```python
from build123d import *

# Parameters (mm, degrees)
SKETCH_R          = 12.75
PAD_DEPTH         = 20
SKETCH001_W       = 2.064916
SKETCH001_H       = 9
POCKET_DEPTH      = 22.001
POCKET_DEPTH_BACK = 22.001


with BuildPart() as part:
    # Sketch → Pad (new body)
    with BuildSketch(Plane.XY):
        with BuildLine():
            ThreePointArc((18.2, -21.818132), (0, 0), (-18.2, -21.818132))
            ThreePointArc((-21.643243, -22.445887), (-19.607744, -23.853631), (-18.2, -21.818132))
            ThreePointArc((-14.264293, -1.750971), (-20.722154, -11.111337), (-21.643243, -22.445887))
            ThreePointArc((-14.264293, -1.750971), (-11.495515, 3.655407), (-13.352959, 9.438568))
            ThreePointArc((13.352959, 9.438568), (0, 38.25), (-13.352959, 9.438568))
            ThreePointArc((13.352959, 9.438568), (11.495515, 3.655407), (14.264293, -1.750971))
            ThreePointArc((21.643243, -22.445887), (20.722154, -11.111337), (14.264293, -1.750971))
            ThreePointArc((18.2, -21.818132), (19.607744, -23.853631), (21.643243, -22.445887))
        make_face()
        with Locations((0, 20.75)):
            Circle(SKETCH_R, mode=Mode.SUBTRACT)
    extrude(amount=PAD_DEPTH)

    # Sketch001 → Pocket (cut, two sides)
    with BuildSketch(Plane.YZ) as pocket_sk:
        with Locations((-20.667451, 10)):
            Rectangle(SKETCH001_W, SKETCH001_H)
    extrude(amount=-POCKET_DEPTH, mode=Mode.SUBTRACT)
    extrude(pocket_sk.sketch, amount=POCKET_DEPTH_BACK, mode=Mode.SUBTRACT)


solid = part.part
```
The listing builds one solid part. Answer for the finished solid, in the listing's coordinates (mm). A direction names the side the tool comes from. Round coordinates to 2 decimals unless told otherwise and drop trailing zeros. Order: outer loops, then holes, each group sorted by start corner. A loop starts at its lowest first (then second) coordinate and runs counter-clockwise, first axis right, second up. Notation, with made-up numbers: (-17, 57) - (26, 57) arc R6 cw to (26, 67) - close; hole circle Ø1 at (-35, 85). An arc over 180 degrees is marked (long way). Put each result on its own line as item: value. Start each with the question number.
(1) Determine the mould class of faces 3 (the cylindrical face through (6.854, 31.501, 9.86)), 4 (the flat face through (-2, 7, 20)), 5 (the flat face through (20, -19.635, 10)) for opening direction Y: released by +Y, released by -Y, zero draft, split by the parting line, or undercut.
(2) Given P1, Ø2, axis at y = 7.5, z = 6.5, coming from the +X side; P2, Ø5, axis at x = -17, z = 14.5, coming from the +Y side; P3, Ø2, axis at x = 6.5, z = 11, coming from the -Y side; P4, Ø2.5, axis at x = 21, y = -21, coming from the -Z side, each flat-ended and moving along its own axis, determine where each tip first touches the part or whether it passes through.
(3) Find section B-B (z = 11.75). Give the vertices of the cut face in (x, y) (3 decimals).
(4) Find section D-D (y = 7). Give the vertices of the cut face in (x, z).
(5) For faces 1 (the flat face through (20, -21, 5.5)), 2 (the cylindrical face through (-11.5, 3.6, 9.9)), determine the directions among +Z, -Z, +X, -X, +Y, -Y from which every point of the face is accessible in a straight line to the end or side of a thin tool.
(6) Straight lines are drawn through the part: probe 1 along X at (y, z) = (-18.5, 10.75); probe 2 along X at (y, z) = (-12, 16); probe 3 along Y at (x, z) = (-9, 14). For each, find the intervals that lie inside material, in ascending order. Write a range as from..to.
(7) Find section A-A (x = 0). Give the vertices of the cut face in (y, z).
(8) Find section C-C (y = -18.5). Give the vertices of the cut face in (x, z).
Reply:
1. face 3: undercut
1. face 4: zero draft
1. face 5: undercut
2. P1: x = 12.67
2. P2: y = 30.55
2. P3: y = -1.59
2. P4: z = 0
3. outline: (-21.971, -19.635) - (-18.465, -19.635) arc R18.5 cw (long way) to (18.465, -19.635) - (21.971, -19.635) arc R22 ccw to (14.264, -1.751) arc R7.949 cw to (13.353, 9.439) arc R17.5 ccw (long way) to (-13.353, 9.439) arc R7.949 cw to (-14.264, -1.751) arc R22 ccw to start; (-21.766, -21.7) arc R22 ccw to (-21.643, -22.446) arc R1.75 ccw to (-18.2, -21.818) arc R18.5 cw to (-18.221, -21.7) - close; (18.2, -21.818) arc R1.75 ccw to (21.643, -22.446) arc R22 ccw to (21.766, -21.7) - (18.221, -21.7) arc R18.5 cw to start; hole circle Ø25.5 at (0, 20.75)
4. outline: (-11.94, 0) - (11.94, 0) - (11.94, 20) - (-11.94, 20) - close
5. face 1: +X, -X
5. face 2: +Z, -Z, -X
6. probe 1: -22..-18.5, 18.5..22
6. probe 2: -21.02..-17.32, 17.32..21.02
6. probe 3: -2.34..11.72, 29.78..35.76
7. outline: (0, 0) - (8, 0) - (8, 20) - (0, 20) - close; (33.5, 0) - (38.25, 0) - (38.25, 20) - (33.5, 20) - close
8. outline: (-22, 0) - (-18.5, 0) - (-18.5, 20) - (-22, 20) - close; (18.5, 0) - (22, 0) - (22, 20) - (18.5, 20) - close
